Verification items for the finished model (mm, model axes). Face numbers are marked on the shaded views. Round coordinates to 2 decimals unless told otherwise and drop trailing zeros. Write item = value, one per line. Start each with the question number.
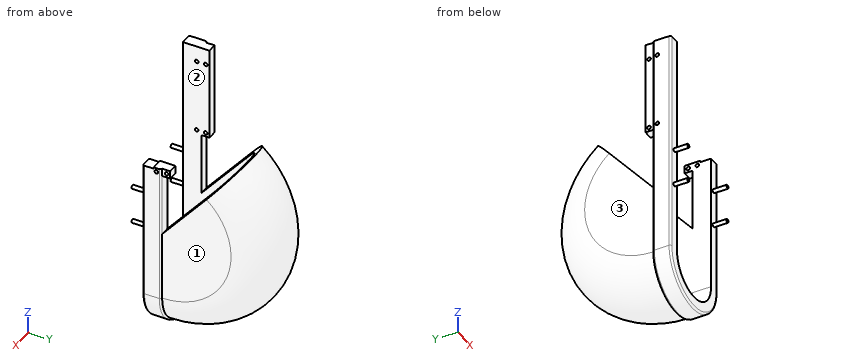
from build123d import *

# Parameters (mm, degrees)
BOSS_EXTRUDE1_DEPTH  = 20
FILLET1_R            = 2
CUT_EXTRUDE3_DEPTH   = 15
REVOLVE1_ANGLE       = 140
CUT_EXTRUDE5_DEPTH   = 20
SKETCH12_R           = 2
BOSS_EXTRUDE3_DEPTH  = 15
SKETCH14_W           = 90
SKETCH14_H           = 51.446942877
CUT_EXTRUDE6_DEPTH   = 10
SKETCH15_R           = 2
BOSS_EXTRUDE4_DEPTH  = 25
SKETCH19_W           = 2
SKETCH19_H           = 5
CUT_EXTRUDE7_DEPTH   = 150
SKETCH21_W           = 90
SKETCH21_H           = 51.374670228
CUT_EXTRUDE9_DEPTH   = 40
CUT_EXTRUDE10_DEPTH  = 20
BOSS_EXTRUDE6_DEPTH  = 1.7
SKETCH28_W           = 10
SKETCH28_H           = 8.8
BOSS_EXTRUDE7_DEPTH  = 7
SKETCH29_W           = 10
SKETCH29_H           = 8.8
BOSS_EXTRUDE8_DEPTH  = 1.7
SKETCH30_R           = 2
CUT_EXTRUDE11_DEPTH  = 89
SKETCH31_W           = 10
SKETCH31_H           = 8.8
BOSS_EXTRUDE9_DEPTH  = 7
SKETCH32_R           = 2
CUT_EXTRUDE12_DEPTH  = 20
SKETCH34_R           = 2
CUT_EXTRUDE13_DEPTH  = 89
SKETCH35_R           = 2
CUT_EXTRUDE14_DEPTH  = 20
BOSS_EXTRUDE10_DEPTH = 95
SKETCH39_R           = 2
CUT_EXTRUDE15_DEPTH  = 80


with BuildPart() as part:
    # Sketch1 → Boss-Extrude1 (new body)
    with BuildSketch(Plane(origin=(0, 0, 0), x_dir=(1, 0, 0), z_dir=(0, 1, 0))):
        with BuildLine():
            Line((0, 0), (0, 150))
            ThreePointArc((0, 150), (-45, 195), (-90, 150))
            Line((-90, 150), (-90, 0))
            ThreePointArc((-90, 0), (-45, -45), (0, 0))
        make_face()
    extrude(amount=-BOSS_EXTRUDE1_DEPTH)

    # Fillet1
    fillet1_edges = [part.edges().sort_by_distance(p)[0] for p in [
        (-45, -20, -195),
        (-90, -20, -75),
        (-45, -20, 45),
        (-90, 0, -75),
        (-45, 0, -195),
        (0, 0, -75),
        (-45, 0, 45),
        (0, -20, -75),
    ]]
    fillet(fillet1_edges, radius=FILLET1_R)

    # Sketch5 → Cut-Extrude3 (cut)
    with BuildSketch(Plane(origin=(0, 0, 0), x_dir=(1, 0, 0), z_dir=(0, 1, 0))):
        with BuildLine():
            Line((-78, 0), (-78, 150))
            ThreePointArc((-78, 150), (-45, 183), (-12, 150))
            Line((-12, 150), (-12, 0))
            ThreePointArc((-12, 0), (-45, -33), (-78, 0))
        make_face()
    extrude(amount=-CUT_EXTRUDE3_DEPTH, mode=Mode.SUBTRACT)

    # Sketch8 → Revolve1 (revolve)
    with BuildSketch(Plane(origin=(0, 0, 0), x_dir=(1, 0, 0), z_dir=(0, 1, 0))):
        with BuildLine():
            Line((-2, 75), (-2, 150))
            ThreePointArc((-2, 150), (-45, 193), (-88, 150))
            Line((-88, 150), (-88, 75))
            Line((-88, 75), (-78, 75))
            Line((-78, 75), (-78, 150))
            ThreePointArc((-78, 150), (-45, 183), (-12, 150))
            Line((-12, 150), (-12, 75))
            Line((-12, 75), (-2, 75))
        make_face()
    revolve(axis=Axis((-12, 0, -75), (1, 0, 0)), revolution_arc=REVOLVE1_ANGLE)

    # Sketch11 → Cut-Extrude5 (cut)
    with BuildSketch(Plane.XZ.offset(20)):
        with BuildLine():
            Line((-76, -150), (-76, 0))
            ThreePointArc((-76, 0), (-45, 31), (-14, 0))
            Line((-14, 0), (-14, -150))
            ThreePointArc((-14, -150), (-45, -181), (-76, -150))
        make_face()
    extrude(amount=-CUT_EXTRUDE5_DEPTH, mode=Mode.SUBTRACT)

    # Sketch12 → Boss-Extrude3 (add)
    with BuildSketch(Plane.XZ.offset(20)):
        with Locations((-83, -75)):
            Circle(SKETCH12_R)
        with Locations((-83, -35)):
            Circle(SKETCH12_R)
        with Locations((-83, 5)):
            Circle(SKETCH12_R)
        with Locations((-7, 5)):
            Circle(SKETCH12_R)
        with Locations((-7, -35)):
            Circle(SKETCH12_R)
        with Locations((-7, -75)):
            Circle(SKETCH12_R)
    extrude(amount=BOSS_EXTRUDE3_DEPTH)

    # Sketch14 → Cut-Extrude6 (cut)
    with BuildSketch(Plane.XZ.offset(20)):
        with Locations((-45, 25.723471439)):
            Rectangle(SKETCH14_W, SKETCH14_H)
    extrude(amount=-CUT_EXTRUDE6_DEPTH, mode=Mode.SUBTRACT)

    # Sketch15 → Boss-Extrude4 (add)
    with BuildSketch(Plane.XZ.offset(35)):
        with Locations((-7, 5)):
            Circle(SKETCH15_R)
        with Locations((-83, 5)):
            Circle(SKETCH15_R)
    extrude(amount=-BOSS_EXTRUDE4_DEPTH)

    # Sketch19 → Cut-Extrude7 (cut)
    with BuildSketch(Plane.XY):
        with Locations((-13, -17.5)):
            Rectangle(SKETCH19_W, SKETCH19_H)
        with Locations((-77, -17.5)):
            Rectangle(SKETCH19_W, SKETCH19_H)
    extrude(amount=-CUT_EXTRUDE7_DEPTH, mode=Mode.SUBTRACT)

    # Sketch21 → Cut-Extrude9 (cut)
    with BuildSketch(Plane(origin=(0, -35, 0), x_dir=(-1, 0, 0), z_dir=(0, -1, 0))):
        with Locations((45, -25.687335114)):
            Rectangle(SKETCH21_W, SKETCH21_H)
    extrude(amount=-CUT_EXTRUDE9_DEPTH, mode=Mode.SUBTRACT)

    # Sketch24 → Cut-Extrude10 (cut)
    with BuildSketch(Plane(origin=(0, -20, 0), x_dir=(-1, 0, 0), z_dir=(0, -1, 0))):
        with BuildLine():
            Line((12, 150), (14, 150))
            ThreePointArc((14, 150), (45, 181), (76, 150))
            Line((76, 150), (78, 150))
            ThreePointArc((78, 150), (45, 183), (12, 150))
        make_face()
    extrude(amount=-CUT_EXTRUDE10_DEPTH, mode=Mode.SUBTRACT)

    # Sketch26 → Boss-Extrude6 (add)
    with BuildSketch(Plane.XY):
        with BuildLine():
            Line((-2, 0), (-12, 0))
            Line((-12, 0), (-12, -8))
            Line((-12, -8), (-2, -8))
            Line((-2, -8), (0, -8))
            Line((0, -8), (0, -2))
            ThreePointArc((0, -2), (-0.585786438, -0.585786438), (-2, 0))
        make_face()
    extrude(amount=BOSS_EXTRUDE6_DEPTH)

    # Sketch28 → Boss-Extrude7 (add)
    with BuildSketch(Plane.XY):
        with Locations((-7, 4.4)):
            Rectangle(SKETCH28_W, SKETCH28_H)
    extrude(amount=-BOSS_EXTRUDE7_DEPTH)

    # Sketch29 → Boss-Extrude8 (add)
    with BuildSketch(Plane.XY):
        with Locations((-7, 4.4)):
            Rectangle(SKETCH29_W, SKETCH29_H)
    extrude(amount=BOSS_EXTRUDE8_DEPTH)

    # Sketch30 → Cut-Extrude11 (cut, through all)
    with BuildSketch(Plane(origin=(-2, 0, 0), x_dir=(0, 0, -1), z_dir=(1, 0, 0))):
        with Locations((2.69, 4.9)):
            Circle(SKETCH30_R)
    extrude(amount=-CUT_EXTRUDE11_DEPTH, mode=Mode.SUBTRACT)

    # Sketch31 → Boss-Extrude9 (add)
    with BuildSketch(Plane.XY):
        with Locations((-83, 4.4)):
            Rectangle(SKETCH31_W, SKETCH31_H)
    extrude(amount=-BOSS_EXTRUDE9_DEPTH)

    # Sketch32 → Cut-Extrude12 (cut)
    with BuildSketch(Plane(origin=(-78, 0, 0), x_dir=(0, 0, -1), z_dir=(1, 0, 0))):
        with Locations((2.69, 4.9)):
            Circle(SKETCH32_R)
    extrude(amount=-CUT_EXTRUDE12_DEPTH, mode=Mode.SUBTRACT)

    # Sketch34 → Cut-Extrude13 (cut, through all)
    with BuildSketch(Plane.ZY.offset(88)):
        with Locations((-2.7, -5.1)):
            Circle(SKETCH34_R)
    extrude(amount=-CUT_EXTRUDE13_DEPTH, mode=Mode.SUBTRACT)

    # Sketch35 → Cut-Extrude14 (cut)
    with BuildSketch(Plane(origin=(-88, 0, 0), x_dir=(0, 0, -1), z_dir=(1, 0, 0))):
        with Locations((2.7, -5.1)):
            Circle(SKETCH35_R)
    extrude(amount=-CUT_EXTRUDE14_DEPTH, mode=Mode.SUBTRACT)

    # Sketch36 → Boss-Extrude10 (add)
    with BuildSketch(Plane.XY):
        with BuildLine():
            Line((-88, -20), (-78, -20))
            Line((-78, -20), (-78, 8.8))
            Line((-78, 8.8), (-88, 8.8))
            Line((-88, 8.8), (-88, 0))
            ThreePointArc((-88, 0), (-89.414213562, -0.585786438), (-90, -2))
            Line((-90, -2), (-90, -18))
            ThreePointArc((-90, -18), (-89.414213562, -19.414213562), (-88, -20))
        make_face()
    extrude(amount=BOSS_EXTRUDE10_DEPTH)

    # Sketch39 → Cut-Extrude15 (cut)
    with BuildSketch(Plane.ZY.offset(90)):
        with Locations((77.5, -5.1)):
            Circle(SKETCH39_R)
        with Locations((77.5, 4.9)):
            Circle(SKETCH39_R)
    extrude(amount=-CUT_EXTRUDE15_DEPTH, mode=Mode.SUBTRACT)


solid = part.part
(1) Scan lines: line 1 along Y through (x, z) = (-80, 77.5); line 2 along Z through (x, y) = (-11, 3.5); line 3 along Y through (x, z) = (-81.75, -2.69). Record each from-to range of solid material in increasing order. Write a range as from..to.
(2) Cross-section at A-A (z = -28). Give the number of separate pieces and of enclosed holes in the cut face, and give its area (3 significant figures).
(3) Depth check by flat-ended pin: pin 1 (1.5 mm diameter, centred on y = 69.5, z = -64, fed in from +X); pin 2 (5 mm diameter, centred on y = -5.1, z = 77.5, fed in from +X); pin 3 (5 mm diameter, centred on y = 14, z = -96.5, fed in from -X); pin 4 (2.5 mm diameter, centred on y = -5.1, z = -2.7, fed in from +X). Enter the tip coordinate at first touch or a pass-through.
(4) Draft check along X on the marked faces 1, 2 and 3. Enter one of: +X half, -X half, draft (parallel to the pull), parting line (faces both ways), or undercut.
Outcome:
q1.line_1 = -20..-7.1, -3.1..2.9, 6.9..8.8
q1.line_2 = -176.26..-70.83, -7..-4.12, -1.26..1.7
q1.line_3 = -20..-7.1, -3.1..2.9, 6.9..8.8, 60.68..65.14
q2.separate_pieces = 3
q2.enclosed_holes = 0
q2.area = 2,230 mm^2
q3.pin_1 = -2
q3.pin_2 = -78
q3.pin_3 = -88
q3.pin_4 = through
q4.face_1 = +X half
q4.face_2 = undercut
q4.face_3 = -X half
